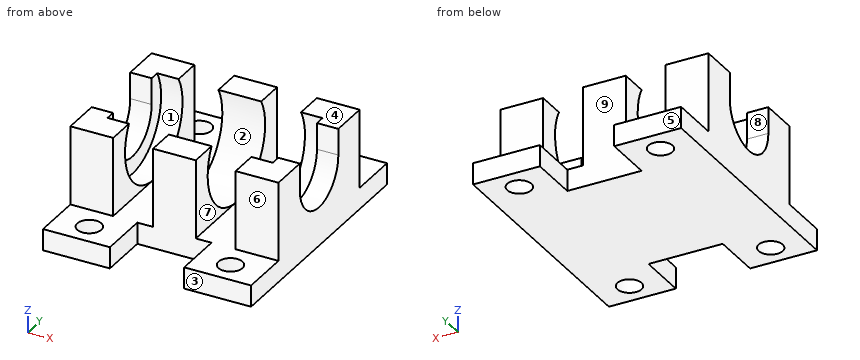
from build123d import *

# Parameters (mm, degrees)
SCHIZZO1_R         = 1.8
BASE_DEPTH         = 3.2
SCHIZZO2_W         = 6.4
SCHIZZO2_H         = 22.1
STAND_OFF_DEPTH    = 11.775
SCHIZZO3_R         = 7.826
BEARING_SLOT_DEPTH = 12.35
SHAFT_HOLES_REACH  = 41.163


with BuildPart() as part:
    # Schizzo1 → Base (new body)
    with BuildSketch(Plane.XY):
        Polygon((-15.55, 11.05), (-15.55, 18.5), (-5.55, 18.5), (-5.55, 11.05), (5.55, 11.05), (5.55, 18.5), (15.55, 18.5), (15.55, 11.05), (15.55, -11.05), (15.55, -18.5), (5.55, -18.5), (5.55, -11.05), (-5.55, -11.05), (-5.55, -18.5), (-15.55, -18.5), (-15.55, -11.05), align=None)
        with Locations((-10.55, 15)):
            Circle(SCHIZZO1_R, mode=Mode.SUBTRACT)
        with Locations(Location((10.55, 15, 0), (0, 0, 180))):
            Circle(SCHIZZO1_R, mode=Mode.SUBTRACT)
        with Locations((10.55, -15)):
            Circle(SCHIZZO1_R, mode=Mode.SUBTRACT)
        with Locations(Location((-10.55, -15, 0), (0, 0, 180))):
            Circle(SCHIZZO1_R, mode=Mode.SUBTRACT)
    extrude(amount=BASE_DEPTH)

    # Schizzo2 → Stand-off (add)
    with BuildSketch(Plane.XY.offset(3.2)):
        with Locations((-12.35, 0)):
            Rectangle(SCHIZZO2_W, SCHIZZO2_H)
        Rectangle(SCHIZZO2_W, SCHIZZO2_H)
        with Locations((12.35, 0)):
            Rectangle(SCHIZZO2_W, SCHIZZO2_H)
    extrude(amount=STAND_OFF_DEPTH)

    # Schizzo3 → Bearing slot (cut, symmetric)
    with BuildSketch(Plane(origin=(0, 0, 0), x_dir=(0, 0, -1), z_dir=(1, 0, 0))):
        with Locations((-11.026, 0)):
            Circle(SCHIZZO3_R)
    extrude(amount=BEARING_SLOT_DEPTH, both=True, mode=Mode.SUBTRACT)

    # Shaft holes: up to this face of the body (flat: up to its plane)
    shaft_holes_end = Plane(part.part.faces().sort_by_distance((15.55, 0, 6.746095849))[0])
    # Schizzo4 → Shaft holes (cut, up to the picked face)
    with BuildSketch(Plane.ZY.offset(15.55), mode=Mode.PRIVATE) as shaft_holes_sk1:
        with BuildLine():
            Line((11.026, 5.25), (14.975, 5.25))
            Line((14.975, 5.25), (14.975, -5.25))
            Line((14.975, -5.25), (11.026, -5.25))
            ThreePointArc((11.026, -5.25), (5.776, 0), (11.026, 5.25))
        make_face()
    shaft_holes_tool1 = split(extrude(shaft_holes_sk1.sketch, amount=-SHAFT_HOLES_REACH, mode=Mode.PRIVATE), bisect_by=shaft_holes_end, keep=Keep.BOTH, mode=Mode.PRIVATE)
    add(shaft_holes_tool1.solids().sort_by(Axis((-15.55, 0, 10.853782), (1, 0, 0)))[0], mode=Mode.SUBTRACT)


solid = part.part
Can you work these out from the model? Positions are in its coordinate system, mm. Face numbers are marked on the shaded views. A direction names the side the tool comes from. Round coordinates to 2 decimals unless told otherwise and drop trailing zeros. Order: outer loops, then holes, each group sorted by start corner. A loop starts at its lowest first (then second) coordinate and runs counter-clockwise, first axis right, second up. Notation, with made-up numbers: (58, 29.25) - (84, 29.25) arc R20 cw to (84, 39.25) - close; hole circle Ø5 at (71.25, 55.5). An arc over 180 degrees is marked (long way). Answer in a Markdown table with one row per item.
(1) Please list where these lines run through material, in increasing order: L1, parallel to Y at x = -10.55, z = 1.05; L2, parallel to X at y = -9, z = 3.75; L3, parallel to X at y = 3, z = 4. Write a range as from..to.
From the geometry:
| item | result |
|---|---|
| L1 | y = -18.5..-16.8, -13.2..13.2, 16.8..18.5 |
| L2 | x = -15.55..-9.15, -3.2..3.2, 9.15..15.55 |
| L3 | x = -15.55..-12.35, 12.35..15.55 |
(2) Suppose I cut it at D-D, the plane y = 10.5. Please give me the cut outline in (x, z) (3 decimals), plus the area to 3 significant figures.
From the geometry:
| item | result |
|---|---|
| outline | (-15.55, 0) - (15.55, 0) - (15.55, 14.975) - (9.15, 14.975) - (9.15, 3.2) - (3.2, 3.2) - (3.2, 14.975) - (-3.2, 14.975) - (-3.2, 3.2) - (-9.15, 3.2) - (-9.15, 14.975) - (-15.55, 14.975) - close |
| area | 326 mm2 |
(3) Which directions (+Z, -Z, +X, -X, +Y, -Y) give clear straight access to the entire face, cutting with the end or side of a thin tool? Please do the marked faces 5, 6, 7, 8 and 9.
From the geometry:
| item | result |
|---|---|
| face 5 | +Z, -Z, +X, -X, +Y |
| face 6 | +Z, +X, -X, -Y |
| face 7 | +Z, +Y, -Y |
| face 8 | +Z, +X, -X |
| face 9 | +Z, -Z, +Y |
(4) Suppose I cut it at A-A, the plane y = -15. Please give me the cut outline in (x, z).
From the geometry:
| item | result |
|---|---|
| outline | (-15.55, 0) - (-12.35, 0) - (-12.35, 3.2) - (-15.55, 3.2) - close; (-8.75, 0) - (-5.55, 0) - (-5.55, 3.2) - (-8.75, 3.2) - close; (5.55, 0) - (8.75, 0) - (8.75, 3.2) - (5.55, 3.2) - close; (12.35, 0) - (15.55, 0) - (15.55, 3.2) - (12.35, 3.2) - close |
(5) If we mould it in two halves opening along Y, with no side actions, what happens to the marked faces 1, 2, 3 and 4? For each: released by +Y, released by -Y, zero draft, split by the parting line, or undercut.
From the geometry:
| item | result |
|---|---|
| face 1 | undercut |
| face 2 | undercut |
| face 3 | released by -Y |
| face 4 | zero draft |
(6) Suppose I cut it at C-C, the plane z = 6.5. Count the separate pieces of the cut face and the enclosed holes in it, plus the area to 3 significant figures.
From the geometry:
| item | result |
|---|---|
| separate pieces | 6 |
| enclosed holes | 0 |
| area | 227 mm2 |
(7) For P1, Ø5, axis at x = 12, z = 10, coming from the +Y side; P2, Ø2.5, axis at x = 14, z = 12.5, coming from the -Y side, each with a flat end and sliding along its axis, tell me the tip position at first contact or that it passes through.
From the geometry:
| item | result |
|---|---|
| P1 | stops at y = 11.05 |
| P2 | stops at y = -11.05 |
(8) Suppose I cut it at B-B, the plane x = 10.55. Please give me the cut outline in (y, z) (3 decimals).
From the geometry:
| item | result |
|---|---|
| outline | (-18.5, 0) - (-16.8, 0) - (-16.8, 3.2) - (-18.5, 3.2) - close; (-13.2, 0) - (13.2, 0) - (13.2, 3.2) - (11.05, 3.2) - (11.05, 14.975) - (6.757, 14.975) arc R7.826 cw (long way) to (-6.757, 14.975) - (-11.05, 14.975) - (-11.05, 3.2) - (-13.2, 3.2) - close; (16.8, 0) - (18.5, 0) - (18.5, 3.2) - (16.8, 3.2) - close |
